Part model, mm, in its own coordinate system. A direction names the side the tool comes from. Coordinates: 2 decimals unless noted, no trailing zeros. Loops run counter-clockwise (first coordinate to the right, second up) from the corner with the lowest first, then second, coordinate; pieces in that order, holes last. Notation, with made-up numbers: (78.5, 59) - (97.5, 59) arc R13 cw to (97.5, 83) - close; hole circle Ø10 at (81, 44.25). An arc over 180 degrees is marked (long way). Use a Markdown table: item, result. Add a question column.
1) Band-saw the part on C-C (x = 14.5). Give the number of separate pieces and of enclosed holes in the cut face, plus the area to 3 significant figures.
2) Band-saw the part on B-B (y = 9.25). Give the cut face in (x, z) (3 decimals), plus the area to 3 significant figures.
3) Probe probe 1 along Y at (x, z) = (0, 1.3); probe 2 along Y at (x, z) = (14.5, 0.65); probe 3 along Z at (x, y) = (10, 4) (3 decimals). List the from-to ranges inside material, lowest first. Write a range as [from, to].
4) Band-saw the part on A-A (x = 0). Give the cut face in (y, z) (3 decimals).
5) Pull direction X, two halves, no side cores. Call faces 1 (the face through (-15.492, 1.767, 1.565)), 2 (the face through (-18, 5, 1)), 3 (the face through (11.846, 10.299, -9.65)), 4 (the face through (0, -2, 0)): +X half, -X half, draft (parallel to the pull), parting line (faces both ways), or undercut.
6) Tool access for faces 5 (the face through (0, 9.693, -6)), 6 (the face through (0, 11, -16)): list every direction of +Z, -Z, +X, -X, +Y, -Y with a clear straight run to the whole face (end or side of a thin tool).
7) Drop flat-ended pins along their axis: P1, Ø1, axis at x = -6, z = -6.5, coming from the -Y side; P2, Ø2, axis at x = 14.5, y = 2.53, coming from the +Z side. Give the stop position or say it passes through.
from build123d import *

# Parameters (mm, degrees)
SKETCH1_W                                            = 36
SKETCH1_H                                            = 21.735371596
SKETCH1_R                                            = 1.25
SKETCH1_R_2                                          = 2.5
SKETCH1_R_3                                          = 1.5
BOSS_EXTRUDE1_DEPTH                                  = 3.175
SKETCH2_W                                            = 36
SKETCH2_H                                            = 3.175
BOSS_EXTRUDE2_DEPTH                                  = 16
SKETCH3_R                                            = 5
SKETCH3_R_2                                          = 2
CUT_EXTRUDE1_DEPTH                                   = 10
ESCAREADO_PARA_PARAFUSO_DE_M_QUINA_COM_C_D           = 4
ESCAREADO_PARA_PARAFUSO_DE_M_QUINA_COM_C_CSINK_D     = 9.4
ESCAREADO_PARA_PARAFUSO_DE_M_QUINA_COM_C_CSINK_ANGLE = 90


with BuildPart() as part:
    # Sketch1 → Boss-Extrude1 (new body)
    with BuildSketch(Plane.XY):
        with Locations((0, 2)):
            Rectangle(SKETCH1_W, SKETCH1_H)
        with Locations((-14.5, 2.527685798)):
            Circle(SKETCH1_R, mode=Mode.SUBTRACT)
        with Locations((14.5, 2.527685798)):
            Circle(SKETCH1_R, mode=Mode.SUBTRACT)
        with Locations((0, 2.527685798)):
            Circle(SKETCH1_R_2, mode=Mode.SUBTRACT)
        with Locations((0, -5.132314202)):
            Circle(SKETCH1_R_3, mode=Mode.SUBTRACT)
    extrude(amount=BOSS_EXTRUDE1_DEPTH)

    # Sketch2 → Boss-Extrude2 (add)
    with BuildSketch(Plane(origin=(0, 0, 0), x_dir=(-1, 0, 0), z_dir=(0, 0, -1))):
        with Locations((0, 11.280185798)):
            Rectangle(SKETCH2_W, SKETCH2_H)
    extrude(amount=BOSS_EXTRUDE2_DEPTH)

    # Sketch3 → Cut-Extrude1 (cut)
    with BuildSketch(Plane.XZ.offset(-9.692685798)):
        with Locations((4.475, -9.744145571)):
            Circle(SKETCH3_R)
        with Locations((-13.025, -4.544145571)):
            Circle(SKETCH3_R_2)
        with Locations((13.975, -9.744145571)):
            Circle(SKETCH3_R_2)
    extrude(amount=-CUT_EXTRUDE1_DEPTH, mode=Mode.SUBTRACT)

    # Escareado para parafuso de máquina com cabeça chata de M42 (through all)
    with Locations(Plane(origin=(0, 12.867685798, 0), x_dir=(-1, 0, 0), z_dir=(0, 1, 0))):
        with Locations((13.025, -4.544145571), (-13.975, -9.744145571)):
            CounterSinkHole(ESCAREADO_PARA_PARAFUSO_DE_M_QUINA_COM_C_D / 2, ESCAREADO_PARA_PARAFUSO_DE_M_QUINA_COM_C_CSINK_D / 2, counter_sink_angle=ESCAREADO_PARA_PARAFUSO_DE_M_QUINA_COM_C_CSINK_ANGLE)


solid = part.part
Answer block:
| question | item | result |
|---|---|---|
| 1 | separate pieces | 3 |
| 1 | enclosed holes | 0 |
| 1 | area | 92.2 mm2 |
| 2 | outline | (-18, 0) - (18, 0) - (18, 3.175) - (-18, 3.175) - close |
| 2 | area | 114 mm2 |
| 3 | probe 1 | [-8.87, -6.63], [-3.63, 0.03], [5.03, 12.87] |
| 3 | probe 2 | [-8.87, 1.28], [3.78, 12.87] |
| 3 | probe 3 | [0, 3.175] |
| 4 | outline | (-8.868, 0) - (-6.632, 0) - (-6.632, 3.175) - (-8.868, 3.175) - close; (-3.632, 0) - (0.028, 0) - (0.028, 3.175) - (-3.632, 3.175) - close; (5.028, 0) - (9.693, 0) - (9.693, -7.514) - (12.868, -7.514) - (12.868, 3.175) - (5.028, 3.175) - close; (9.693, -16) - (12.868, -16) - (12.868, -11.974) - (9.693, -11.974) - close |
| 5 | face 1 | undercut |
| 5 | face 2 | -X half |
| 5 | face 3 | undercut |
| 5 | face 4 | draft |
| 6 | face 5 | -Z, +X, -X, -Y |
| 6 | face 6 | -Z, +X, -X, +Y, -Y |
| 7 | P1 | y = 9.69 |
| 7 | P2 | through |
